For this review, take the finished solid that the model builds, in its own axes (mm). A direction names the side the tool comes from. Give positions to 0.01 mm unless a question says otherwise; leave off trailing zeros. Loops run counter-clockwise (first coordinate to the right, second up) from the corner with the lowest first, then second, coordinate; pieces in that order, holes last. Notation, with made-up numbers: (-33.5, 88) - (25.5, 88) arc R20 cw to (25.5, 119) - close; hole circle Ø10 at (-19.5, 56). An arc over 180 degrees is marked (long way). Put each result on its own line as item: value.
from build123d import *

# Parameters (mm, degrees)
SKETCH1_R           = 2
SKETCH1_W           = 43
SKETCH1_H           = 43
BOSS_EXTRUDE1_DEPTH = 7
SKETCH2_W           = 43
SKETCH2_H           = 43
SKETCH2_R           = 12.5
SKETCH2_R_2         = 1.55
BOSS_EXTRUDE2_DEPTH = 2
SKETCH3_W           = 51
SKETCH3_H           = 51
SKETCH3_W_2         = 43
SKETCH3_H_2         = 43
BOSS_EXTRUDE3_DEPTH = 4
SKETCH4_R           = 5.15
CUT_EXTRUDE1_DEPTH  = 2
SKETCH5_R           = 1.85
CUT_EXTRUDE2_DEPTH  = 10


with BuildPart() as part:
    # Sketch1 → Boss-Extrude1 (new body)
    with BuildSketch(Plane(origin=(0, 0, 0), x_dir=(1, 0, 0), z_dir=(0, 1, 0))):
        with BuildLine():
            Line((-132.651439051, 63.421561199), (54.631829022, 63.421561199))
            ThreePointArc((54.631829022, 63.421561199), (58.167362928, 61.957095105), (59.631829022, 58.421561199))
            Line((59.631829022, 58.421561199), (59.631829022, -59.578438801))
            ThreePointArc((59.631829022, -59.578438801), (58.167362928, -63.113972707), (54.631829022, -64.578438801))
            Line((54.631829022, -64.578438801), (-132.651439051, -64.578438801))
            ThreePointArc((-132.651439051, -64.578438801), (-136.186972957, -63.113972707), (-137.651439051, -59.578438801))
            Line((-137.651439051, -59.578438801), (-137.651439051, 58.421561199))
            ThreePointArc((-137.651439051, 58.421561199), (-136.186972957, 61.957095105), (-132.651439051, 63.421561199))
        make_face()
        with Locations((-132.651439051, 58.421561199)):
            Circle(SKETCH1_R, mode=Mode.SUBTRACT)
        with Locations((54.631829022, -59.578438801)):
            Circle(SKETCH1_R, mode=Mode.SUBTRACT)
        with Locations((29.631829022, 49.421561199)):
            Circle(SKETCH1_R, mode=Mode.SUBTRACT)
        with Locations((-15.368170978, 49.421561199)):
            Circle(SKETCH1_R, mode=Mode.SUBTRACT)
        with Locations((-107.651439051, -50.578438801)):
            Circle(SKETCH1_R, mode=Mode.SUBTRACT)
        with Locations((-62.651439051, -50.578438801)):
            Circle(SKETCH1_R, mode=Mode.SUBTRACT)
        with Locations((-91.151439051, 16.921561199)):
            Rectangle(SKETCH1_W, SKETCH1_H, mode=Mode.SUBTRACT)
        with Locations((13.131829022, -18.078438801)):
            Rectangle(SKETCH1_W, SKETCH1_H, mode=Mode.SUBTRACT)
    extrude(amount=BOSS_EXTRUDE1_DEPTH)

    # Sketch2 → Boss-Extrude2 (add)
    with BuildSketch(Plane(origin=(0, 7, 0), x_dir=(1, 0, 0), z_dir=(0, 1, 0))):
        with Locations((-91.151439051, 16.921561199)):
            Rectangle(SKETCH2_W, SKETCH2_H)
        with Locations((-91.151439051, 16.921561199)):
            Circle(SKETCH2_R, mode=Mode.SUBTRACT)
        with Locations((-106.651439051, 32.421561199)):
            Circle(SKETCH2_R_2, mode=Mode.SUBTRACT)
        with Locations((-75.651439051, 32.421561199)):
            Circle(SKETCH2_R_2, mode=Mode.SUBTRACT)
        with Locations((-75.651439051, 1.421561199)):
            Circle(SKETCH2_R_2, mode=Mode.SUBTRACT)
        with Locations((-106.651439051, 1.421561199)):
            Circle(SKETCH2_R_2, mode=Mode.SUBTRACT)
        with Locations((13.131829022, -18.078438801)):
            Rectangle(SKETCH2_W, SKETCH2_H)
        with Locations((13.131829022, -18.078438801)):
            Circle(SKETCH2_R, mode=Mode.SUBTRACT)
        with Locations((28.631829022, -33.578438801)):
            Circle(SKETCH2_R_2, mode=Mode.SUBTRACT)
        with Locations((-2.368170978, -33.578438801)):
            Circle(SKETCH2_R_2, mode=Mode.SUBTRACT)
        with Locations((-2.368170978, -2.578438801)):
            Circle(SKETCH2_R_2, mode=Mode.SUBTRACT)
        with Locations((28.631829022, -2.578438801)):
            Circle(SKETCH2_R_2, mode=Mode.SUBTRACT)
    extrude(amount=-BOSS_EXTRUDE2_DEPTH)

    # Sketch3 → Boss-Extrude3 (add)
    with BuildSketch(Plane.XZ):
        with Locations((13.131829022, 18.078438801)):
            Rectangle(SKETCH3_W, SKETCH3_H)
        with Locations((13.131829022, 18.078438801)):
            Rectangle(SKETCH3_W_2, SKETCH3_H_2, mode=Mode.SUBTRACT)
        with Locations((-91.151439051, -16.921561199)):
            Rectangle(SKETCH3_W, SKETCH3_H)
        with Locations((-91.151439051, -16.921561199)):
            Rectangle(SKETCH3_W_2, SKETCH3_H_2, mode=Mode.SUBTRACT)
    extrude(amount=BOSS_EXTRUDE3_DEPTH)

    # Sketch4 → Cut-Extrude1 (cut)
    with BuildSketch(Plane(origin=(0, 7, 0), x_dir=(1, 0, 0), z_dir=(0, 1, 0))):
        with Locations((-132.651439051, 58.421561199)):
            Circle(SKETCH4_R)
        with Locations((-15.368170978, 49.421561199)):
            Circle(SKETCH4_R)
        with Locations((29.631829022, 49.421561199)):
            Circle(SKETCH4_R)
        with Locations((54.631829022, -59.578438801)):
            Circle(SKETCH4_R)
        with Locations((-62.651439051, -50.578438801)):
            Circle(SKETCH4_R)
        with Locations((-107.651439051, -50.578438801)):
            Circle(SKETCH4_R)
    extrude(amount=-CUT_EXTRUDE1_DEPTH, mode=Mode.SUBTRACT)

    # Sketch5 → Cut-Extrude2 (cut)
    with BuildSketch(Plane.XZ):
        with Locations((-116.651439051, 33.49401297)):
            Circle(SKETCH5_R)
        with Locations((-27.651439051, 33.49401297)):
            Circle(SKETCH5_R)
        with Locations((-50.368170978, -32.337135367)):
            Circle(SKETCH5_R)
        with Locations((38.631829022, -32.337135367)):
            Circle(SKETCH5_R)
    extrude(amount=-CUT_EXTRUDE2_DEPTH, mode=Mode.SUBTRACT)


solid = part.part
1) Insertion check: pin 1 Ø1.2 at (y, z) = (-2.5, -15) entering from -X; pin 2 Ø6 at (x, z) = (-50.37, -32.34) entering from -Y; pin 3 Ø3.5 at (x, z) = (-116.65, 33.49) entering from +Y; pin 4 Ø5 at (x, z) = (-14, -51) entering from +Y. Each pin has a flat end and moves straight along its axis. Give the tip position at first contact, or say it passes through.
Geometry check:
pin 1: stops at x = -116.65
pin 2: stops at y = 0
pin 3: passes through
pin 4: stops at y = 5
2) Take a section at B-B on z = -25.5. State the section outline as (x, y) points.
Geometry check:
outline: (-137.65, 0) - (-116.65, 0) - (-116.65, -4) - (-112.65, -4) - (-112.65, 5) - (-100.24, 5) - (-100.24, 7) - (-137.65, 7) - close; (-82.06, 5) - (-69.65, 5) - (-69.65, -4) - (-65.65, -4) - (-65.65, 0) - (59.63, 0) - (59.63, 7) - (-82.06, 7) - close
3) Take a section at A-A on x = -88. State the section outline as (y, z) points, and give its area (3 significant figures).
Geometry check:
outline: (-4, -42.42) - (0, -42.42) - (0, -63.42) - (7, -63.42) - (7, -29.02) - (5, -29.02) - (5, -38.42) - (-4, -38.42) - close; (-4, 4.58) - (5, 4.58) - (5, -4.83) - (7, -4.83) - (7, 64.58) - (0, 64.58) - (0, 8.58) - (-4, 8.58) - close
area: 665 mm²
4) Draft analysis for pull direction Z (two halves, no side actions). For faces 5 (the face through (13, 1, 39.578)), 6 (the face through (-40, 3, -63.422)), 7 (the face through (-12.368, -2, 18)), state which applies: pulls with the +Z half, pulls with the -Z half, needs draft (parallel to the pull), parting line crosses it, or undercut.
Geometry check:
face 5: undercut
face 6: pulls with the -Z half
face 7: needs draft
5) For faces 1 (the face through (-91, 1, -38.422)), 2 (the face through (-92, -2, 8.578)), 3 (the face through (-130, 5, -58)), 4 (the face through (-65.651, -2, -17)), list the 3-axis set-ups (+Z, -Z, +X, -X, +Y, -Y) from which the entire face can be reached by the end or side of a thin tool; tool diameter is ignored.
Geometry check:
face 1: -Y
face 2: +Z, -X, -Y
face 3: +Y
face 4: +Z, -Z, -Y
6) Wall thickness on line 1 (Z direction, x = 18, y = 0.75); line 2 (Z direction, x = -71.5, y = -2); line 3 (X direction, y = 2, z = -13): over which ranges is each line inside the solid? List them lowest first.
Geometry check:
line 1: z = -63.42 to -3.42, 39.58 to 64.58
line 2: z = -42.42 to -38.42, 4.58 to 8.58
line 3: x = -137.65 to -112.65, -69.65 to 59.63
